The listing builds one solid part. Answer for the finished solid, in the listing's coordinates (mm). A direction names the side the tool comes from. Round coordinates to 2 decimals unless told otherwise and drop trailing zeros. Write each loop counter-clockwise with the first axis right and the second up, starting at its lowest first coordinate (ties: lowest second). Pieces come first, ordered by that corner, then holes.
Item 1: Find section B-B on x = 8. Give the vertices of the cut face in (y, z), then the cut area to 3 significant figures.
Item 2: For a pull along Z with two mould halves and no side action, classify faces 3 (the face through (26.9, 3.8, 2.7)), 4 (the face through (37.57, -1.38, -6.2)), 5 (the face through (0, 3, 0)) as +Z half, -Z half, draft (parallel to the pull), parting line (faces both ways), or undercut.
Item 3: Find section A-A on z = 0. Give the vertices of the cut face in (x, y) (3 decimals), then the cut area to 3 significant figures.
Item 4: Find section C-C on z = -4.25. Give the vertices of the cut face in (x, y), then the cut area to 3 significant figures.
Item 5: Each of these flat-tipped pins is pushed along its axis until it touches: pin 1 (7.5 mm diameter, centred on y = 0, z = 0, fed in from -X); pin 2 (4 mm diameter, centred on x = 48, z = -5, fed in from -Y); pin 3 (5 mm diameter, centred on x = 16, z = -3, fed in from +Y); pin 4 (3 mm diameter, centred on x = 31, z = 4.5, fed in from +Y). Where does it stop, or does it pass through?
Item 6: Find the intervals of material crossed by probe 1 along Z at (x, y) = (18.5, 0) (3 decimals); probe 2 along Z at (x, y) = (8, 0); probe 3 along X at (y, z) = (4, 0), in increasing order.
Item 7: A tool of negligible diameter and unlimited length cuts with its end or side. For faces 1 (the face through (57.417, -0.661, 5.037)), 2 (the face through (6.44, -0.5, -2.23)), from which of +Z, -Z, +X, -X, +Y, -Y can it reach the whole face along a straight path? Write none if from no direction.
Item 8: Find section D-D on x = 66.5. Give the vertices of the cut face in (y, z).
```python
from build123d import *

# Parameters (mm, degrees)
F0_R     = 6.35
F1_DEPTH = 76.2
F2_R     = 5.08
F3_DEPTH = 38.1
F4_R     = 3.175
F5_DEPTH = 25.4
F6_R     = 2.286
F7_DEPTH = 25.4
F8_R     = 3.175
F9_DEPTH = 25.4


with BuildPart() as f1:
    # F0 (on Right) → F1 (new body)
    with BuildSketch(Plane.YZ):
        Circle(F0_R)
    extrude(amount=F1_DEPTH)

    # F2 (on face) → F3 (cut)
    with BuildSketch(Plane.YZ.offset(76.2)):
        Circle(F2_R)
    extrude(amount=-F3_DEPTH, mode=Mode.SUBTRACT)

    # F4 (on face) → F5 (cut)
    with BuildSketch(Plane.YZ.offset(38.1)):
        Circle(F4_R)
    extrude(amount=-F5_DEPTH, mode=Mode.SUBTRACT)

    # F6 (on face) → F7 (cut)
    with BuildSketch(Plane.YZ.offset(12.7)):
        Circle(F6_R)
    extrude(amount=-F7_DEPTH, mode=Mode.SUBTRACT)

    # F8 (on Front) → F9 (cut)
    with BuildSketch(Plane.XZ):
        with Locations((25.229068, 0)):
            Circle(F8_R)
    extrude(amount=-F9_DEPTH, mode=Mode.SUBTRACT)


solid = f1.part
```
Check values:
1. outline: circle Ø12.7 at (0, 0); hole circle Ø4.57 at (0, 0)
1. area: 110 mm2
2. face 3: undercut
2. face 4: parting line
2. face 5: draft
3. outline: (0, -6.35) - (76.2, -6.35) - (76.2, -5.08) - (38.1, -5.08) - (38.1, -3.175) - (12.7, -3.175) - (12.7, -2.286) - (0, -2.286) - close; (0, 2.286) - (12.7, 2.286) - (12.7, 3.175) - (22.054, 3.175) - (22.054, 6.35) - (0, 6.35) - close; (28.404, 3.175) - (38.1, 3.175) - (38.1, 5.08) - (76.2, 5.08) - (76.2, 6.35) - (28.404, 6.35) - close
3. area: 341 mm2
4. outline: (0, -4.72) - (76.2, -4.72) - (76.2, -2.78) - (38.1, -2.78) - (38.1, 2.78) - (76.2, 2.78) - (76.2, 4.72) - (0, 4.72) - close
4. area: 507 mm2
5. pin 1: stops at x = 0
5. pin 2: stops at y = -5.6
5. pin 3: stops at y = 6.33
5. pin 4: stops at y = 5.6
6. probe 1: z = -6.35 to -3.175, 3.175 to 6.35
6. probe 2: z = -6.35 to -2.29, 2.29 to 6.35
6. probe 3: x = 0 to 22.05, 28.4 to 38.1
7. face 1: +X
7. face 2: +X, -X
8. outline: circle Ø12.7 at (0, 0); hole circle Ø10.16 at (0, 0)
